Input: part model. Units: mm. Frame: model coordinates. Coordinates: 2 decimals unless noted, no trailing zeros. Order: outer loops, then holes, each group sorted by start corner. A loop starts at its lowest first (then second) coordinate and runs counter-clockwise, first axis right, second up. Notation, with made-up numbers: (51.25, 27) - (82.25, 27) arc R29 cw to (82.25, 57) - close; hole circle Ø4 at (73.25, 26.5). An arc over 180 degrees is marked (long way). One line per question, with ' | ' between items. Start each with the question number.
Autodesk Inventor part; units mm, degrees
ref_plane "YZ Plane" through (0, 0, 0) normal (1, 0, 0) x (0, 1, 0)
ref_plane "XZ Plane" through (0, 0, 0) normal (0, 1, 0) x (-1, 0, 0)
ref_plane "XY Plane" through (0, 0, 0) normal (0, 0, 1) x (1, 0, 0)
sketch "Sketch1" plane through (0, 0, 0) normal (0, 0, 1) x (1, 0, 0)
  circle A0 centre (0, 0) radius 3.9497
  dimension "d0" = 7.8994
extrude "Extrusion1" add sketch "Sketch1" against normal mid plane 130.175
sketch "Sketch2" plane through (0, 0, 0) normal (0, 1, 0) x (-1, 0, 0)
  circle A0 centre (0, 61.9125) radius 1.3208
  line L0 (-3.9497, 65.0875) -> (3.9497, 65.0875)
  point P0 (0, 65.0875)
  dimension "d3" = 2.6416
  dimension "d4" = 3.175
extrude "Extrusion2" cut sketch "Sketch2" along normal through all both and the other way through all
mirror "Mirror1" about plane through (0, 0, 0) normal (0, 0, 1) of "Extrusion2"
properties part number "Handle_Rod" material "Steel, Mild"
(1) Section A-A (x = 0). Output: boundary loops of the cut face in (y, z).
(2) Draft query along Z for faces 1 (the face through (0, 0, -65.088)), 2 (the face through (0, 0, 65.088)), 3 (the face through (0.286, -0.055, -60.623)). Return one class per face: +Z half, -Z half, draft (parallel to the pull), parting line (faces both ways), or undercut.
(3) Material intervals for line 1 along Z through (x, y) = (0, 2); line 2 along Z through (x, y) = (0.5, 3) (1 decimal); line 3 along X through (y, z) = (-0.25, -51.5), sorted ascending. Write a range as from..to.
(4) Section C-C (z = -44). Output: boundary loops of the cut face in (x, y), then the cut area to 3 significant figures.
(5) Pin query (flat end, axial travel): pin 1 (2 mm diameter, centred on x = 0, z = -61.91, fed in from -Y); pin 2 (2 mm diameter, centred on y = -2, z = -30.5, fed in from +X). Return the tip coordinate at first contact, or that it passes through.
(6) Section B-B (y = 2.5). Output: boundary loops of the cut face in (x, z), then the cut area to 3 significant figures.
Worked answers:
1) outline: (-3.95, -65.09) - (3.95, -65.09) - (3.95, -63.23) - (-3.95, -63.23) - close; (-3.95, -60.59) - (3.95, -60.59) - (3.95, 60.59) - (-3.95, 60.59) - close; (-3.95, 63.23) - (3.95, 63.23) - (3.95, 65.09) - (-3.95, 65.09) - close
2) face 1: -Z half | face 2: +Z half | face 3: undercut
3) line 1: z = -65.09..-63.23, -60.59..60.59, 63.23..65.09 | line 2: z = -65.1..-63.1, -60.7..60.7, 63.1..65.1 | line 3: x = -3.94..3.94
4) outline: circle Ø7.9 at (0, 0) | area: 49.0 mm²
5) pin 1: passes through | pin 2: stops at x = 3.82
6) outline: (-3.06, -65.09) - (3.06, -65.09) - (3.06, 65.09) - (-3.06, 65.09) - close; hole circle Ø2.64 at (0, -61.91); hole circle Ø2.64 at (0, 61.91) | area: 785 mm²
